CAD build for the part. Positions are in the model's coordinates, mm. A direction names the side the tool comes from. Give positions to 0.01 mm unless a question says otherwise; leave off trailing zeros. Write each loop counter-clockwise with the first axis right and the second up, starting at its lowest first coordinate (ties: lowest second). Pieces come first, ordered by that corner, then holes. Notation, with made-up numbers: M -7.5,-14.75 L 39.5,-14.75 A27 ccw 39.5,2.25 Z; hole C 30,-29 d3. An arc over 180 degrees is marked long. One line per question, with ' | ' between items. Start each with the question number.
1. Cut at A-A, the plane x = -11. Write the cut outline in (y, z), then the cut area to 3 significant figures.
2. Cut at C-C, the plane z = 1.6. Count the separate pieces of the cut face and the enclosed holes in it, then the cut area to 3 significant figures.
3. Cut at B-B, the plane y = 79. Write the cut outline in (x, z).
4. Flat gauge pins, fed straight in: pin 1 (1.5 mm diameter, centred on y = -4.5, z = 2, fed in from +X); pin 2 (2 mm diameter, centred on x = -34, y = 15.5, fed in from -Z); pin 3 (1.5 mm diameter, centred on x = -68.5, z = 2, fed in from -Y); pin 4 (0.9 mm diameter, centred on x = 11.5, z = 2, fed in from +Y). Where does each tip first touch, or does it go through?
5. Wall check: L1, parallel to Y at x = -23, z = 2; L2, parallel to X at y = 49.5, z = 1.15; L3, parallel to Y at x = -11, z = 2.45. Give the ranges that are in metal, low to high.
6. Which spindle directions (+Z, -Z, +X, -X, +Y, -Y) get a long thin tool onto all of the face, cutting with end or side? Do faces 4 (the face through (2.006, 149, 1)), 5 (the face through (-63, 147.603, 1)), 6 (the face through (-49.394, 70, 2)), 7 (the face through (2.006, -4, 1)), 8 (the face through (-47.994, -4, 1)). Say none if no direction does.
7. Cut at D-D, the plane x = -26.5. Write the cut outline in (y, z).
8. Pull direction Y, two halves, no side cores. Call faces 1 (the face through (32.006, 72, 1)), 2 (the face through (1.606, 71, 2)), 3 (the face through (17, -2.397, 1)): released by +Y, released by -Y, zero draft, split by the parting line, or undercut.
Autodesk Inventor part; units mm, degrees
ref_plane "YZ Plane" through (0, 0, 0) normal (1, 0, 0) x (0, 1, 0)
ref_plane "XZ Plane" through (0, 0, 0) normal (0, 1, 0) x (-1, 0, 0)
ref_plane "XY Plane" through (0, 0, 0) normal (0, 0, 1) x (1, 0, 0)
sketch "Sketch1" plane through (0, 0, 0) normal (0, 0, 1) x (1, 0, 0)
  line L0 (-77.994, -2.3973) -> (-47.994, -2.3973)
  line L1 (-47.994, -2.3973) -> (-47.994, -5.3973)
  line L2 (-47.994, -5.3973) -> (2.006, -5.3973)
  line L3 (2.006, -2.3973) -> (32.006, -2.3973)
  line L4 (32.006, -2.3973) -> (32.006, 147.6027)
  line L5 (32.006, 147.6027) -> (2.006, 147.6027)
  line L6 (2.006, 147.6027) -> (2.006, 150.6027)
  line L7 (2.006, 150.6027) -> (-47.994, 150.6027)
  line L8 (-47.994, 150.6027) -> (-47.994, 147.6027)
  line L9 (-47.994, 147.6027) -> (-77.994, 147.6027)
  line L10 (2.006, -2.3973) -> (2.006, -5.3973)
  line L11 (-77.994, 147.6027) -> (-77.994, -2.3973)
  point P0 (0, 0)
  dimension "d0" = 150
  dimension "d1" = 3
  dimension "d2" = 3
  dimension "d3" = 50
  dimension "d4" = 50
  dimension "d5" = 30
  dimension "d6" = 30
extrude "Extrusion1" add sketch "Sketch1" along normal blind 3
sketch "Sketch2" plane through (0, 0, 3) normal (0, 0, 1) x (1, 0, 0)
  line L0 (27.506, 96.0027) -> (27.506, 98.7027)
  line L1 (-77.994, 147.6027) -> (-77.994, -2.3973)
  circle A0 centre (24.806, 49.2027) radius 1.75
  circle A1 centre (24.806, 96.0027) radius 1.75
  circle A2 centre (-61.194, 96.0027) radius 1.75
  circle A3 centre (-61.194, 49.2027) radius 1.75
  line L2 (27.506, 50.6827) -> (27.506, 46.5027)
  line L3 (1.606, 50.6827) -> (-49.394, 50.6827)
  line L4 (-49.394, 50.6827) -> (-49.394, 90.6827)
  line L5 (-49.394, 90.6827) -> (1.606, 90.6827)
  line L6 (1.606, 90.6827) -> (1.606, 50.6827)
  line L7 (32.006, 147.6027) -> (2.006, 147.6027)
  point P0 (0, 0)
extrude "Extrusion2" cut sketch "Sketch2" against normal blind 3
sketch "Sketch3" plane through (0, 0, 3) normal (0, 0, 1) x (1, 0, 0)
  circle A0 centre (-61.194, 49.2027) radius 1.75
  point P0 (0, 0)
sketch "Sketch4" plane through (0, 0, 3) normal (0, 0, 1) x (1, 0, 0)
  circle A0 centre (-61.194, 96.0027) radius 1.75
  line L0 (-77.994, 147.6027) -> (-77.994, -2.3973)
  circle A1 centre (-50.494, 123.146) radius 6.5
  circle A2 centre (-22.994, 123.146) radius 6.5
  circle A3 centre (4.506, 123.146) radius 6.5
  point P0 (0, 0)
  point P1 (32.006, 147.6027)
  dimension "d48" = 13
  dimension "d49" = 13
  dimension "d50" = 13
extrude "Extrusion3" cut sketch "Sketch4" against normal blind 3 contours A1 | A2 | A3
properties part number "test"
Here are the results:
1) outline: M -5.4,0 L 50.68,0 L 50.68,3 L -5.4,3 Z; M 90.68,0 L 150.6,0 L 150.6,3 L 90.68,3 Z | area: 348 mm^2
2) separate pieces: 1 | enclosed holes: 8 | area: 14,300 mm^2
3) outline: M -77.99,0 L -49.39,0 L -49.39,3 L -77.99,3 Z; M 1.61,0 L 32.01,0 L 32.01,3 L 1.61,3 Z
4) pin 1: x = 2.01 | pin 2: z = 0 | pin 3: y = -2.4 | pin 4: y = 147.6
5) L1: -5.4 to 50.68, 90.68 to 116.65, 129.65 to 150.6 | L2: -77.99 to -62.92, -59.47 to 23.08, 26.53 to 32.01 | L3: -5.4 to 50.68, 90.68 to 150.6
6) face 4: +Z, -Z, +X, +Y | face 5: +Z, -Z, -X, +Y | face 6: +Z, -Z | face 7: +Z, -Z, +X, -Y | face 8: +Z, -Z, -X, -Y
7) outline: M -5.4,0 L 50.68,0 L 50.68,3 L -5.4,3 Z; M 90.68,0 L 117.67,0 L 117.67,3 L 90.68,3 Z; M 128.62,0 L 150.6,0 L 150.6,3 L 128.62,3 Z
8) face 1: zero draft | face 2: undercut | face 3: released by -Y
